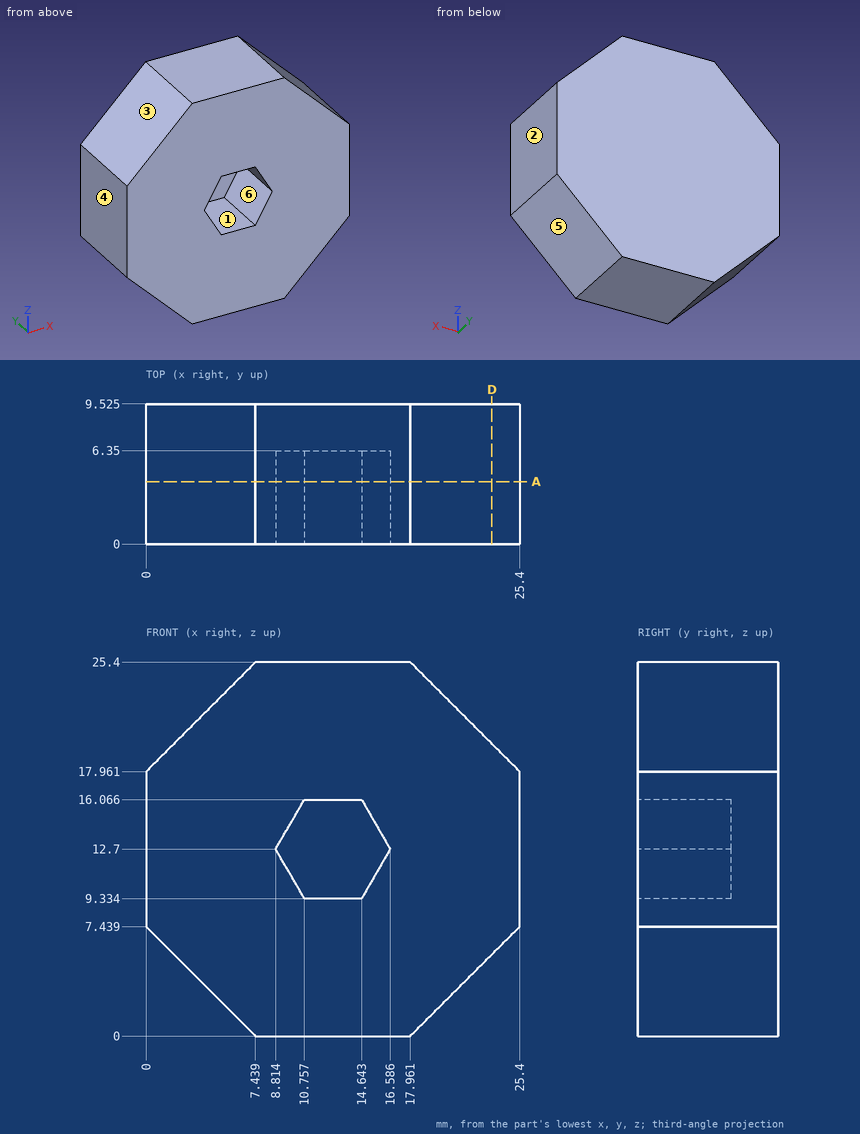
Design review of the part shown in the three views and the two pictorial views. Dimensions are in mm from the part's minimum x, y and z. A direction names the side the tool comes from. Give positions to 0.01 mm unless a question says otherwise; leave off trailing zeros. Write each loop counter-clockwise with the first axis right and the second up, starting at its lowest first coordinate (ties: lowest second). Pieces come first, ordered by that corner, then holes. Notation, with made-up numbers: M 42.5,55.5 L 96.5,55.5 A28 cw 96.5,75.5 Z; hole C -26.75,24 d7. An arc over 180 degrees is marked long. One line per question, with ' | ' between items. Start each with the question number.
Item 1: Draft analysis for pull direction Z (two halves, no side actions). For the marked faces 3, 4, 5 and 6, state which applies: released by +Z, released by -Z, zero draft, split by the parting line, or undercut.
Item 2: For the marked faces 1 and 2, list the 3-axis set-ups (+Z, -Z, +X, -X, +Y, -Y) from which the entire face can be reached by the end or side of a thin tool; tool diameter is ignored.
Item 3: We need section D-D on x = 23.5. Write out the cut boundary in (y, z) (1 decimal).
Item 4: We need section A-A on y = 4.25. Write out the cut boundary in (x, z) (1 decimal), plus the area to 3 significant figures.
Item 5: Wall thickness on line 1 (Z direction, x = 14.25, y = 4.75) (1 decimal); line 2 (X direction, y = 1.25, z = 12.75); line 3 (X direction, y = 5.75, z = 4.75): over which ranges is each line inside the solid? List them lowest first. Write a range as from..to.
Item 6: For pin 1 (1 mm diameter, centred on x = 4, y = 3, fed in from +Z); pin 2 (3.5 mm diameter, centred on x = 12, z = 13.5, fed in from -Y); pin 3 (3 mm diameter, centred on x = 22.5, y = 3, fed in from -Z), all flat-tipped, find the tip position at first contact; note any pin that passes through.
Results found:
1) face 3: released by +Z | face 4: zero draft | face 5: released by -Z | face 6: undercut
2) face 1: -Y | face 2: +Z, -Z, +X, +Y, -Y
3) outline: M 0,5.5 L 9.5,5.5 L 9.5,19.9 L 0,19.9 Z
4) outline: M 0,7.4 L 7.4,0 L 18,0 L 25.4,7.4 L 25.4,18 L 18,25.4 L 7.4,25.4 L 0,18 Z; hole M 8.8,12.7 L 10.8,9.3 L 14.6,9.3 L 16.6,12.7 L 14.6,16.1 L 10.8,16.1 Z | area: 495 mm2
5) line 1: z = 0..9.3, 16.1..25.4 | line 2: x = 0..8.84, 16.56..25.4 | line 3: x = 2.69..22.71
6) pin 1: stops at z = 22.46 | pin 2: stops at y = 6.35 | pin 3: stops at z = 3.04
